Here's how the part is built. I have some questions about the finished solid (model axes, mm). A direction names the side the tool comes from. Coordinates: 2 decimals unless noted, no trailing zeros. Loops run counter-clockwise (first coordinate to the right, second up) from the corner with the lowest first, then second, coordinate; pieces in that order, holes last. Notation, with made-up numbers: M 85,-7 L 123,-7 A30 cw 123,22 Z; hole C 12.5,-34 d3. An arc over 180 degrees is marked long. Use CSV: the item, a comma, the result in double quotes. Start each with the question number.
Q1. If we section it at A-A (z = -247): Please give me the cut outline in (x, y), and give its area (3 significant figures).
Q2. If we mould it in two halves opening along X, with no side actions, what happens to faces 1 (the flat face through (965.2, 508, -213)), 2 (the flat face through (508, 965.2, -213)), 3 (the flat face through (482.6, 26, -213))? For each: +X half, -X half, draft (parallel to the pull), parting line (faces both ways), or undercut.
Q3. Which directions (+Z, -Z, +X, -X, +Y, -Y) give clear straight access to the entire face, cutting with the end or side of a thin tool? Please do faces 4 (the flat face through (533.4, 991, -213)), 5 (the flat face through (991, 482.6, -213)), 6 (the flat face through (508, 50.8, -213)), 7 (the flat face through (482.6, 991, -213)), 8 (the flat face through (990, 533.4, -213)).
Q4. If we section it at B-B (y = 343): Please give me the cut outline in (x, z).
Q5. Please list where this line runs through material, in increasing order: probe 1 along Z at (x, y) = (240.5, 796.5). Write a range as [from, to].
Q6. For pin 1 Ø15 at (x, z) = (37.5, -222.5) entering from -Y; pin 2 Ø15 at (x, z) = (20.5, -298) entering from +Y; pin 3 Ø6 at (x, y) = (665.5, 736) entering from -Z, each with a flat end and sliding along its axis, tell me the tip position at first contact or that it passes through.
from build123d import *

# Parameters (mm, degrees)
F0_W     = 1016
F0_H     = 1016
F1_DEPTH = 25.4
F2_W     = 50.8
F2_H     = 50.8
F3_DEPTH = 431.8


with BuildPart() as f1:
    # F0 (on Top) → F1 (new body)
    with BuildSketch(Plane.XY):
        with Locations((508, 508)):
            Rectangle(F0_W, F0_H)
    extrude(amount=F1_DEPTH)

    # F2 (on face) → F3 (join)
    with BuildSketch(Plane(origin=(0, 0, 0), x_dir=(1, 0, 0), z_dir=(0, 0, -1))):
        Polygon((50.8, -482.6), (0, -482.6), (0, -508), (0, -533.4), (50.8, -533.4), align=None)
        Polygon((1016, -533.4), (1016, -508), (1016, -482.6), (965.2, -482.6), (965.2, -533.4), align=None)
        with Locations((508, -990.6)):
            Rectangle(F2_W, F2_H)
        with Locations((508, -25.4)):
            Rectangle(F2_W, F2_H)
    extrude(amount=F3_DEPTH)


solid = f1.part
Results below:
1,outline,"M 0,482.6 L 50.8,482.6 L 50.8,533.4 L 0,533.4 Z; M 482.6,0 L 533.4,0 L 533.4,50.8 L 482.6,50.8 Z; M 482.6,965.2 L 533.4,965.2 L 533.4,1016 L 482.6,1016 Z; M 965.2,482.6 L 1016,482.6 L 1016,533.4 L 965.2,533.4 Z"
1,area,"10,300 mm^2"
2,face 1,"undercut"
2,face 2,"draft"
2,face 3,"-X half"
3,face 4,"-Z, +X, +Y, -Y"
3,face 5,"-Z, +X, -X, -Y"
3,face 6,"-Z, +X, -X"
3,face 7,"-Z, -X, +Y, -Y"
3,face 8,"-Z, +X, -X, +Y"
4,outline,"M 0,0 L 1016,0 L 1016,25.4 L 0,25.4 Z"
5,probe 1,"[0, 25.4]"
6,pin 1,"y = 482.6"
6,pin 2,"y = 533.4"
6,pin 3,"z = 0"
